Check sheet for the modelled part. Datum: model origin and axes. Units: mm. A direction names the side the tool comes from. Coordinates: 2 decimals unless noted, no trailing zeros. Order: outer loops, then holes, each group sorted by start corner. A loop starts at its lowest first (then second) coordinate and runs counter-clockwise, first axis right, second up.
from build123d import *

# Parameters (mm, degrees)
F0_R     = 2.5
F2_DEPTH = 0.7
F3_DEPTH = 0.8


# Not quite as in the source:
# - a fillet or chamfer that OpenCascade refuses, or shapes differently, is made with other operations: its cross-section is extruded or revolved along the edge and cut away or added


with BuildPart() as f2:
    # F0 (on Front) → F2 (new body, symmetric)
    with BuildSketch(Plane.XZ):
        Circle(F0_R)
        with BuildLine():
            ThreePointArc((0, 1.6670872347), (1.1788086885, 1.1788086885), (1.6670872347, 0))
            ThreePointArc((1.6670872347, 0), (1.1788086885, -1.1788086885), (0, -1.6670872347))
            ThreePointArc((0, -1.6670872347), (-1.1788086885, -1.1788086885), (-1.6670872347, 0))
            ThreePointArc((-1.6670872347, 0), (-1.1788086885, 1.1788086885), (0, 1.6670872347))
        make_face(mode=Mode.SUBTRACT)
        Polygon((1.035158575, 0), (0, 1.6670872347), (-1.035158575, 0), (0, -1.6670872347), align=None)
        with BuildLine():
            Line((1.035158575, 0), (1.6670872347, 0))
            ThreePointArc((1.6670872347, 0), (1.1788086885, 1.1788086885), (0, 1.6670872347))
            Line((0, 1.6670872347), (1.035158575, 0))
        make_face()
        with BuildLine():
            ThreePointArc((-1.6670872347, 0), (-1.1788086885, -1.1788086885), (0, -1.6670872347))
            Line((0, -1.6670872347), (-1.035158575, 0))
            Line((-1.035158575, 0), (-1.6670872347, 0))
        make_face()
    extrude(amount=F2_DEPTH, both=True)

    # F1 (on Right) → F3 (join, symmetric)
    with BuildSketch(Plane.YZ):
        Polygon((4.6792123099, 0), (0, 0), (4.6792123099, -0.7401879564), (6.3069890554, -3.2957927736), (6.3069890554, -4.3182368269), (6.3069890554, -5.7057410895), (6.9458728476, -5.7057410895), (6.9458728476, -4.3182368269), (6.9458728476, -3.2957927736), align=None)
    extrude(amount=F3_DEPTH, both=True)

    # F4: fillet of radius 1.2553910524 on 1 edges, made by hand

    # F4_s1 → F4_t2 (revolve, cut)
    with BuildSketch(Plane.XY):
        with BuildLine():
            ThreePointArc((2.5, 0.5553910524), (2.1323044738, -0.3323044738), (1.2446089476, -0.7))
            Line((1.2446089476, -0.7), (2.5, -0.7))
            Line((2.5, -0.7), (2.5, 0.5553910524))
        make_face()
    revolve(axis=Axis((0, -0.7, 0), (0, -1, 0)), mode=Mode.SUBTRACT)


solid = f2.part
(1) Cross-section at B-B (y = 6.5). Enter the section's corners in (x, z), and give its area (3 significant figures).
Filled in:
outline: (-0.8, -5.71) - (0.8, -5.71) - (0.8, -2.65) - (-0.8, -2.65) - close
area: 4.89 mm2
(2) Release check for a two-part mould opening along Z. For faces 6 (the flat face through (-0.51, -0.01, 0.845)), 7 (the flat face through (0.01, 2.66, -0.42)), 8 (the flat face through (-0.8, 5.43, -1.57)) record: +Z half, -Z half, draft (parallel to the pull), parting line (faces both ways), or undercut.
Filled in:
face 6: undercut
face 7: -Z half
face 8: draft
(3) Go/stop test with flat-tipped pins: P1, Ø1, axis at x = 0.5, y = 3, coming from the +Z side; P2, Ø3, axis at y = 4.5, z = -2.5, coming from the +X side; P3, Ø0.5, axis at x = -0.5, z = -4.5, coming from the -Y side; P4, Ø2, axis at x = -2, z = -3.5, coming from the +Y side. Record where each tip stops, or that it passes through.
Filled in:
P1: stops at z = 0
P2: stops at x = 0.8
P3: stops at y = 6.31
P4: passes through
(4) Tool access check on faces 1 (the flat face through (0.8, 5.43, -1.57)), 2 (the flat face through (0, 3, 0)), 3 (the flat face through (0.01, 5.48, -2)), 4 (the flat face through (0, -0.7, 0)), 5 (the flat face through (0, 6.307, -4)). Record the directions out of +Z, -Z, +X, -X, +Y, -Y that give a thin tool (end or side, any length) a straight path to the whole face; none if there is none.
Filled in:
face 1: +Z, -Z, +X, +Y
face 2: +Z, +X, -X, +Y
face 3: -Z, +X, -X
face 4: +Z, -Z, +X, -X, -Y
face 5: -Z, +X, -X, -Y
(5) Cross-section at A-A (z = -3.75). Enter the section's corners in (x, y).
Filled in:
outline: (-0.8, 6.31) - (0.8, 6.31) - (0.8, 6.95) - (-0.8, 6.95) - close
(6) Thickness scan on probe 1 along Y at (x, z) = (-0.3, -3.75); probe 2 along X at (y, z) = (6.5, -4.5); probe 3 along Z at (x, y) = (0.75, 5.75). Record the ranges inside material, lowest first.
Filled in:
probe 1: y = 6.31 to 6.95
probe 2: x = -0.8 to 0.8
probe 3: z = -2.42 to -1.56
